CAD build for the part. Positions are in the model's coordinates, mm. Round coordinates to 2 decimals unless told otherwise and drop trailing zeros. Write each loop counter-clockwise with the first axis right and the second up, starting at its lowest first coordinate (ties: lowest second). Pieces come first, ordered by that corner, then holes. Notation, with made-up numbers: (9.25, 19) - (25.25, 19) arc R12 ccw to (25.25, 40) - close; hole circle Ø2 at (26, 32). An arc over 180 degrees is marked (long way). Put each result on its own line as item: value. Start each with the question number.
Item 1: Drill centre lines: line 1 (Z direction, x = 10, y = 1.55); line 2 (Z direction, x = -17, y = 1.45); line 3 (X direction, y = 3.6, z = -17.5). Where is each one in solid material? Low to high. Write a range as from..to.
Item 2: Cut at C-C (y = 0.9). Count the separate pieces of the cut face and the enclosed holes in it, and give its area (3 significant figures).
Item 3: Cut at A-A (x = 25). Give the cut face in (y, z).
Item 4: Cut at B-B (z = -35). Give the cut face in (x, y).
Item 5: Cut at D-D (z = -11). Give the cut face in (x, y), and give its area (3 significant figures).
Item 6: Pin check, flat tips, straight feed: pin 1 Ø5.5 at (x, z) = (-17.68, 17.68) entering from +Y; pin 2 Ø2 at (y, z) = (3.5, 10) entering from -X; pin 3 Ø1.5 at (x, y) = (-11.5, 2) entering from +Z; pin 4 Ø2.5 at (x, z) = (0, -25) entering from +Y. Stop position of each tip, or through.
```python
from build123d import *

# Parameters (mm, degrees)
SKETCH_1_R      = 40
SKETCH_1_R_2    = 2.15
SKETCH_1_R_3    = 1.65
EXTRUDE_2_DEPTH = 5


with BuildPart() as part:
    # 草图1 → 凸台-拉伸2 (new body)
    with BuildSketch(Plane(origin=(0, 0, 0), x_dir=(1, 0, 0), z_dir=(0, 1, 0))):
        with Locations(Location((0, 0, 0), (0, 0, 270))):
            Circle(SKETCH_1_R)
        with Locations(Location((0, 35, 0), (0, 0, 270))):
            Circle(SKETCH_1_R_2, mode=Mode.SUBTRACT)
        with Locations(Location((30.310889132, 17.5, 0), (0, 0, 270))):
            Circle(SKETCH_1_R_2, mode=Mode.SUBTRACT)
        with Locations(Location((30.310889132, -17.5, 0), (0, 0, 270))):
            Circle(SKETCH_1_R_2, mode=Mode.SUBTRACT)
        with Locations(Location((0, -35, 0), (0, 0, 270))):
            Circle(SKETCH_1_R_2, mode=Mode.SUBTRACT)
        with Locations(Location((-30.310889132, -17.5, 0), (0, 0, 270))):
            Circle(SKETCH_1_R_2, mode=Mode.SUBTRACT)
        with Locations(Location((-30.310889132, 17.5, 0), (0, 0, 270))):
            Circle(SKETCH_1_R_2, mode=Mode.SUBTRACT)
        with Locations(Location((0, 25, 0), (0, 0, 270))):
            Circle(SKETCH_1_R_2, mode=Mode.SUBTRACT)
        with Locations(Location((17.67766953, 17.67766953, 0), (0, 0, 270))):
            Circle(SKETCH_1_R_2, mode=Mode.SUBTRACT)
        with Locations(Location((25, 0, 0), (0, 0, 270))):
            Circle(SKETCH_1_R_2, mode=Mode.SUBTRACT)
        with Locations(Location((17.67766953, -17.67766953, 0), (0, 0, 270))):
            Circle(SKETCH_1_R_2, mode=Mode.SUBTRACT)
        with Locations(Location((0, -25, 0), (0, 0, 270))):
            Circle(SKETCH_1_R_2, mode=Mode.SUBTRACT)
        with Locations(Location((-17.67766953, -17.67766953, 0), (0, 0, 270))):
            Circle(SKETCH_1_R_2, mode=Mode.SUBTRACT)
        with Locations(Location((-25, 0, 0), (0, 0, 270))):
            Circle(SKETCH_1_R_2, mode=Mode.SUBTRACT)
        with Locations(Location((-17.67766953, 17.67766953, 0), (0, 0, 270))):
            Circle(SKETCH_1_R_2, mode=Mode.SUBTRACT)
        with Locations(Location((0, 15, 0), (0, 0, 270))):
            Circle(SKETCH_1_R_3, mode=Mode.SUBTRACT)
        with Locations(Location((10.606601718, 10.606601718, 0), (0, 0, 270))):
            Circle(SKETCH_1_R_3, mode=Mode.SUBTRACT)
        with Locations(Location((15, 0, 0), (0, 0, 270))):
            Circle(SKETCH_1_R_3, mode=Mode.SUBTRACT)
        with Locations(Location((10.606601718, -10.606601718, 0), (0, 0, 270))):
            Circle(SKETCH_1_R_3, mode=Mode.SUBTRACT)
        with Locations(Location((0, -15, 0), (0, 0, 270))):
            Circle(SKETCH_1_R_3, mode=Mode.SUBTRACT)
        with Locations(Location((-10.606601718, -10.606601718, 0), (0, 0, 270))):
            Circle(SKETCH_1_R_3, mode=Mode.SUBTRACT)
        with Locations(Location((-15, 0, 0), (0, 0, 270))):
            Circle(SKETCH_1_R_3, mode=Mode.SUBTRACT)
        with Locations(Location((-10.606601718, 10.606601718, 0), (0, 0, 270))):
            Circle(SKETCH_1_R_3, mode=Mode.SUBTRACT)
    extrude(amount=EXTRUDE_2_DEPTH)


solid = part.part
```
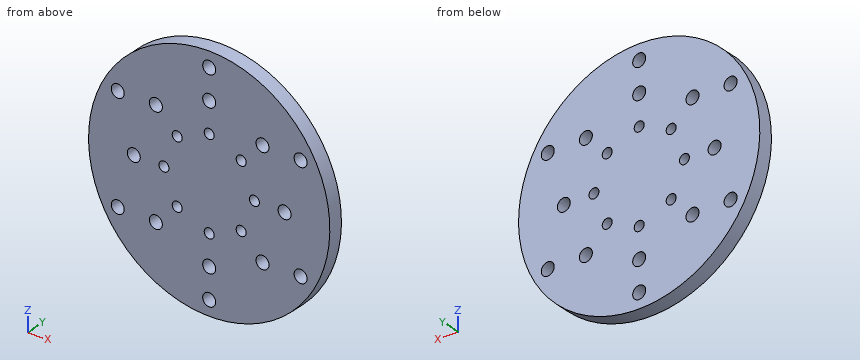
Output values:
1. line 1: -38.73..-12.14, -9.07..9.07, 12.14..38.73
1. line 2: -36.21..-19.72, -15.64..15.64, 19.72..36.21
1. line 3: -35.97..-32.46, -28.16..-19.82, -15.54..15.54, 19.82..28.16, 32.46..35.97
2. separate pieces: 1
2. enclosed holes: 22
2. area: 4,750 mm2
3. outline: (0, -31.22) - (5, -31.22) - (5, -2.15) - (0, -2.15) - close; (0, 2.15) - (5, 2.15) - (5, 31.22) - (0, 31.22) - close
4. outline: (-19.36, 0) - (-2.15, 0) - (-2.15, 5) - (-19.36, 5) - close; (2.15, 0) - (19.36, 0) - (19.36, 5) - (2.15, 5) - close
5. outline: (-38.46, 0) - (-12.21, 0) - (-12.21, 5) - (-38.46, 5) - close; (-9, 0) - (9, 0) - (9, 5) - (-9, 5) - close; (12.21, 0) - (38.46, 0) - (38.46, 5) - (12.21, 5) - close
5. area: 353 mm2
6. pin 1: y = 5
6. pin 2: x = -38.97
6. pin 3: z = 38.53
6. pin 4: through
